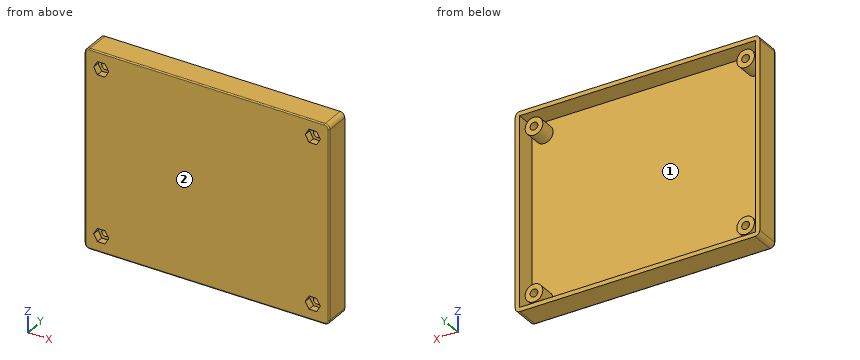
```python
from build123d import *

# Parameters (mm, degrees)
ESQUISSE1_W             = 104
ESQUISSE1_H             = 84
BOSS_EXTRU_1_DEPTH      = 2
ESQUISSE2_R             = 3.75
BOSS_EXTRU_2_DEPTH      = 7
ESQUISSE3_W             = 104
ESQUISSE3_H             = 84
ESQUISSE3_W_2           = 100.4
ESQUISSE3_H_2           = 80.4
BOSS_EXTRU_3_DEPTH      = 8.55
ESQUISSE4_R             = 1.65
ENL_V_MAT_EXTRU_1_DEPTH = 68.446274916
ENL_V_MAT_EXTRU_2_DEPTH = 3
CONG_1_R                = 2
CONG_2_R                = 0.5


with BuildPart() as part:
    # Esquisse1 → Boss.-Extru.1 (new body)
    with BuildSketch(Plane(origin=(0, 0, 0), x_dir=(1, 0, 0), z_dir=(0, 1, 0))):
        Rectangle(ESQUISSE1_W, ESQUISSE1_H)
    extrude(amount=BOSS_EXTRU_1_DEPTH)

    # Esquisse2 → Boss.-Extru.2 (add)
    with BuildSketch(Plane(origin=(0, 2, 0), x_dir=(1, 0, 0), z_dir=(0, 1, 0))):
        with Locations(Location((-45, 35, 0), (0, 0, 270))):
            Circle(ESQUISSE2_R)
        with Locations(Location((45, 35, 0), (0, 0, 270))):
            Circle(ESQUISSE2_R)
        with Locations(Location((45, -35, 0), (0, 0, 270))):
            Circle(ESQUISSE2_R)
        with Locations(Location((-45, -35, 0), (0, 0, 270))):
            Circle(ESQUISSE2_R)
    extrude(amount=BOSS_EXTRU_2_DEPTH)

    # Esquisse3 → Boss.-Extru.3 (add)
    with BuildSketch(Plane(origin=(0, 2, 0), x_dir=(1, 0, 0), z_dir=(0, 1, 0))):
        Rectangle(ESQUISSE3_W, ESQUISSE3_H)
        Rectangle(ESQUISSE3_W_2, ESQUISSE3_H_2, mode=Mode.SUBTRACT)
    extrude(amount=BOSS_EXTRU_3_DEPTH)

    # Esquisse4 → Enlèv. mat.-Extru.1 (cut, through all)
    with BuildSketch(Plane(origin=(0, 9, 0), x_dir=(1, 0, 0), z_dir=(0, 1, 0))):
        with Locations(Location((-45, 35, 0), (0, 0, 270))):
            Circle(ESQUISSE4_R)
        with Locations(Location((45, 35, 0), (0, 0, 270))):
            Circle(ESQUISSE4_R)
        with Locations(Location((45, -35, 0), (0, 0, 270))):
            Circle(ESQUISSE4_R)
        with Locations(Location((-45, -35, 0), (0, 0, 270))):
            Circle(ESQUISSE4_R)
    extrude(amount=-ENL_V_MAT_EXTRU_1_DEPTH, mode=Mode.SUBTRACT)

    # Esquisse5 → Enlèv. mat.-Extru.2 (cut)
    with BuildSketch(Plane.XZ):
        Polygon((-43.397853003, 32.225), (-41.795706006, 35), (-43.397853003, 37.775), (-46.602146997, 37.775), (-48.204293994, 35), (-46.602146997, 32.225), align=None)
        Polygon((43.397853003, 32.225), (46.602146997, 32.225), (48.204293994, 35), (46.602146997, 37.775), (43.397853003, 37.775), (41.795706006, 35), align=None)
        Polygon((43.397853003, -32.225), (41.795706006, -35), (43.397853003, -37.775), (46.602146997, -37.775), (48.204293994, -35), (46.602146997, -32.225), align=None)
        Polygon((-46.602146997, -32.225), (-48.204293994, -35), (-46.602146997, -37.775), (-43.397853003, -37.775), (-41.795706006, -35), (-43.397853003, -32.225), align=None)
    extrude(amount=-ENL_V_MAT_EXTRU_2_DEPTH, mode=Mode.SUBTRACT)

    # Congé1
    cong_1_edges = [part.edges().sort_by_distance(p)[0] for p in [
        (-52, 5.275, -42),
        (52, 5.275, -42),
        (52, 5.275, 42),
        (-52, 5.275, 42),
    ]]
    fillet(cong_1_edges, radius=CONG_1_R)

    # Congé2
    cong_2_edges = [part.edges().sort_by_distance(p)[0] for p in [
        (-52, 0, 0),
        (0, 0, -42),
        (52, 0, 0),
        (0, 0, 42),
        (51.414213562, 0, 41.414213562),
        (51.414213562, 0, -41.414213562),
        (-51.414213562, 0, 41.414213562),
        (-51.414213562, 0, -41.414213562),
    ]]
    fillet(cong_2_edges, radius=CONG_2_R)


solid = part.part
```
Source: CAD feature listing. Evaluate the final solid. Frame: model axes, mm. Face numbers are marked on the shaded views. Round coordinates to 2 decimals unless told otherwise and drop trailing zeros. Order: outer loops, then holes, each group sorted by start corner. A loop starts at its lowest first (then second) coordinate and runs counter-clockwise, first axis right, second up. Notation, with made-up numbers: (-21.75, 51) -> (15.25, 51) arc R26 ccw to (15.25, 81) -> close; hole circle Ø1 at (-23.5, 38). An arc over 180 degrees is marked (long way). Use CSV: the item, a comma, the result in double quotes.
(1) Pull-direction query (X, two-part tool) for the marked faces 1 and 2; classes: +X half, -X half, draft (parallel to the pull), parting line (faces both ways), or undercut.
Report:
face 1,"undercut"
face 2,"draft"
(2) Ray query, L1, parallel to X at y = 5.65, z = 35; L2, parallel to Z at x = 44.5, y = 1 (3 decimals); L3, parallel to Z at x = 10, y = 4.25. Return the intervals inside material, ascending.
Report:
L1,"-52 to -50.2, -48.75 to -46.65, -43.35 to -41.25, 41.25 to 43.35, 46.65 to 48.75, 50.2 to 52"
L2,"-42 to -37.775, -32.225 to 32.225, 37.775 to 42"
L3,"-42 to -40.2, 40.2 to 42"
(3) Section D-D on x = 34. Return the cut outline in (y, z).
Report:
outline,"(0, -41.5) arc R0.5 ccw to (0.5, -42) -> (10.55, -42) -> (10.55, -40.2) -> (2, -40.2) -> (2, 40.2) -> (10.55, 40.2) -> (10.55, 42) -> (0.5, 42) arc R0.5 ccw to (0, 41.5) -> close"
(4) Section A-A on y = 6.25. Count the separate pieces of the cut face and the enclosed holes in it, and give its area (3 significant figures).
Report:
separate pieces,"5"
enclosed holes,"5"
area,"803 mm^2"
(5) Section C-C on z = 2. Return the cut outline in (x, y), and give its area (3 significant figures).
Report:
outline,"(-52, 0.5) arc R0.5 ccw to (-51.5, 0) -> (51.5, 0) arc R0.5 ccw to (52, 0.5) -> (52, 10.55) -> (50.2, 10.55) -> (50.2, 2) -> (-50.2, 2) -> (-50.2, 10.55) -> (-52, 10.55) -> close"
area,"239 mm^2"
(6) First-contact query: pin 1 Ø4.5 at (x, z) = (-45, -35) entering from +Y; pin 2 Ø3 at (x, z) = (-44.5, -35.5) entering from -Y. Flat tips, straight axial feed; report the tip coordinate or a pass-through.
Report:
pin 1,"y = 9"
pin 2,"y = 3"
